Geometry check sheet. Reference: the model listing, model coordinates, mm. Round coordinates to 2 decimals unless told otherwise and drop trailing zeros. Loops run counter-clockwise (first coordinate to the right, second up) from the corner with the lowest first, then second, coordinate; pieces in that order, holes last. Notation, with made-up numbers: M -28,76.5 L -17,76.5 A10 ccw -17,82.5 Z; hole C 28,62.5 d7. An arc over 180 degrees is marked long. Use one line per item in the form item = value. Start each with the question number.
1. Cross-section at D-D (x = -19.05). Record the boundary of the cut face in (y, z) (3 decimals), then the cut area to 3 significant figures.
2. Cross-section at A-A (z = 0). Record the boundary of the cut face in (x, y) (3 decimals), then the cut area to 3 significant figures.
3. Cross-section at C-C (y = 20.75). Record the boundary of the cut face in (x, z) (3 decimals).
4. Cross-section at B-B (x = 0). Record the boundary of the cut face in (y, z) (3 decimals), then the cut area to 3 significant figures.
5. Material ranges on line 1 (X direction, y = 16, z = 38.1) (3 decimals); line 2 (Z direction, x = -19.05, y = 12) (3 decimals); line 3 (Z direction, x = 0, y = 9.25) (3 decimals), recorded low to high.
Autodesk Inventor part; units mm, degrees
ref_plane "YZ Plane" through (0, 0, 0) normal (1, 0, 0) x (0, 1, 0)
ref_plane "XZ Plane" through (0, 0, 0) normal (0, 1, 0) x (-1, 0, 0)
ref_plane "XY Plane" through (0, 0, 0) normal (0, 0, 1) x (1, 0, 0)
sketch "Sketch2" plane through (0, 0, 0) normal (0, 1, 0) x (-1, 0, 0)
  line L0 (-44.45, 50.8) -> (44.45, 50.8)
  line L1 (44.45, 50.8) -> (44.45, -50.8)
  line L2 (44.45, -50.8) -> (-44.45, -50.8)
  line L3 (-44.45, -50.8) -> (-44.45, 50.8)
  point P0 (0, 0)
  dimension "d0" = 44.45
  dimension "d1" = 44.45
  dimension "d2" = 50.8
  dimension "d3" = 50.8
extrude "Extrusion1" add sketch "Sketch2" along normal blind 25.4
fillet "Fillet1" radius 12.7 4 edges at (44.45, 12.7, 50.8) (-44.45, 12.7, 50.8) (44.45, 12.7, -50.8) (-44.45, 12.7, -50.8)
sketch "Sketch3" plane through (0, 25.4, 0) normal (0, 1, 0) x (1, 0, 0)
  line L0 (-44.45, -38.1) -> (-44.45, 38.1)
  line L1 (31.75, -50.8) -> (-31.75, -50.8)
  line L2 (44.45, 38.1) -> (44.45, -38.1)
  line L3 (-31.75, 50.8) -> (31.75, 50.8)
  point P0 (0, 0)
  point P1 (-19.05, 38.1)
  point P2 (19.05, 38.1)
  point P3 (19.05, -38.1)
  point P4 (-19.05, -38.1)
  point P5 (0, 0)
  dimension "d7" = 25.4
  dimension "d8" = 25.4
  dimension "d9" = 12.7
  dimension "d10" = 12.7
hole "Hole1" at (-19.05, 25.4, -38.1) at (19.05, 25.4, -38.1) at (19.05, 25.4, 38.1) at (-19.05, 25.4, 38.1) at (0, 25.4, 0) direction (0, -1, 0) diameter 6.35 end through all
properties part number "Fixed Extension" material "Aluminum-6061"
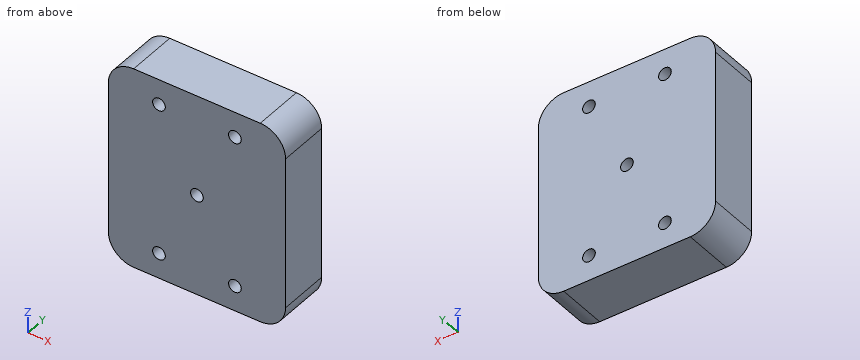
Reported:
q1.outline = M 0,-50.8 L 25.4,-50.8 L 25.4,-41.275 L 0,-41.275 Z; M 0,-34.925 L 25.4,-34.925 L 25.4,34.925 L 0,34.925 Z; M 0,41.275 L 25.4,41.275 L 25.4,50.8 L 0,50.8 Z
q1.area = 2,260 mm²
q2.outline = M -44.45,0 L -3.175,0 L -3.175,25.4 L -44.45,25.4 Z; M 3.175,0 L 44.45,0 L 44.45,25.4 L 3.175,25.4 Z
q2.area = 2,100 mm²
q3.outline = M -44.45,-38.1 A12.7 ccw -31.75,-50.8 L 31.75,-50.8 A12.7 ccw 44.45,-38.1 L 44.45,38.1 A12.7 ccw 31.75,50.8 L -31.75,50.8 A12.7 ccw -44.45,38.1 Z; hole C -19.05,-38.1 d6.35; hole C -19.05,38.1 d6.35; hole C 0,0 d6.35; hole C 19.05,-38.1 d6.35; hole C 19.05,38.1 d6.35
q4.outline = M 0,-50.8 L 25.4,-50.8 L 25.4,-3.175 L 0,-3.175 Z; M 0,3.175 L 25.4,3.175 L 25.4,50.8 L 0,50.8 Z
q4.area = 2,420 mm²
q5.line_1 = -44.45 to -22.225, -15.875 to 15.875, 22.225 to 44.45
q5.line_2 = -50.8 to -41.275, -34.925 to 34.925, 41.275 to 50.8
q5.line_3 = -50.8 to -3.175, 3.175 to 50.8
